from build123d import *

# Parameters (mm, degrees)
SKETCH_1_W           = 28
SKETCH_1_H           = 16
EXTRUDE_1_DEPTH      = 2
EXTRUDE_2_DEPTH      = 2
FILLET_1_R           = 3
SKETCH_3_R           = 1
CUT_EXTRUDE_1_DEPTH  = 34.526109228
EXTRUDE_3_DEPTH      = 1
EXTRUDE_3_DEPTH_BACK = 25
SKETCH_5_R           = 1
SKETCH_6_R           = 2
SKETCH_6_R_2         = 5
CUT_EXTRUDE_2_DEPTH  = 2


with BuildPart() as part:
    # Sketch 1 → Extrude 1 (new body)
    with BuildSketch(Plane(origin=(0, 0, 0), x_dir=(1, 0, 0), z_dir=(0, 1, 0))):
        Rectangle(SKETCH_1_W, SKETCH_1_H)
    extrude(amount=EXTRUDE_1_DEPTH)

    # Sketch 2 → Extrude 2 (add)
    with BuildSketch(Plane.ZY.offset(14)):
        Polygon((-8, 0), (-8, 2), (1, 12), (14, 12), (14, 6), (8, 6), (8, 2), (8, 0), align=None)
    extrude_2 = extrude(amount=-EXTRUDE_2_DEPTH)

    # Mirror 1: Extrude 2 across plane
    add(extrude_2.mirror(Plane(origin=(0, 0, 0), x_dir=(0, 0, 1), z_dir=(1, 0, 0))))

    # Fillet 1
    fillet_1_edges = [part.edges().sort_by_distance(p)[0] for p in [
        (13, 6, 14),
        (13, 12, 14),
        (-13, 6, 14),
        (-13, 12, 14),
    ]]
    fillet(fillet_1_edges, radius=FILLET_1_R - 0.0001)  # a hair under: the kernel refuses the full size

    # Sketch 3 → Cut-Extrude 1 (cut, through all)
    with BuildSketch(Plane.ZY.offset(14)):
        with Locations((11, 9)):
            Circle(SKETCH_3_R)
    extrude(amount=-CUT_EXTRUDE_1_DEPTH, mode=Mode.SUBTRACT)



with BuildPart() as body_2:
    # Sketch 4 → Revolve 2 (revolve)
    with BuildSketch(Plane(origin=(0, 9, 0), x_dir=(1, 0, 0), z_dir=(0, 1, 0))):
        with BuildLine():
            Line((-11.75, -11), (-11.75, -13.5))
            Line((-11.75, -13.5), (-3.056178347, -17.553995615))
            ThreePointArc((-3.056178347, -17.553995615), (0, -18.231534043), (3.056178347, -17.553995615))
            Line((3.056178347, -17.553995615), (11.75, -13.5))
            Line((11.75, -13.5), (11.75, -11))
            Line((11.75, -11), (-11.75, -11))
        make_face()
    revolve(axis=Axis((14, 9, 11), (-1, 0, 0)))


with BuildPart() as part_1:
    add(part.part)

    add(body_2.part)  # Extrude 3 merges body 2
    # Sketch 5 → Extrude 3 (add, two sides: drawn at the far end of the back side and taken through both)
    with BuildSketch(Plane(origin=(11.75, 0, 0), x_dir=(0, 0, -1), z_dir=(1, 0, 0)).offset(-EXTRUDE_3_DEPTH_BACK)):
        with Locations(Location((-11, 9, 0), (0, 0, 180))):
            Circle(SKETCH_5_R)
    extrude(amount=EXTRUDE_3_DEPTH + EXTRUDE_3_DEPTH_BACK)

    # Sketch 6 → Cut-Extrude 2 (cut)
    with BuildSketch(Plane.XZ):
        with Locations(Location((-8, 2, 0), (0, 0, 270))):
            Circle(SKETCH_6_R)
        with Locations(Location((8, 2, 0), (0, 0, 270))):
            Circle(SKETCH_6_R)
        with Locations(Location((0, 2, 0), (0, 0, 270))):
            Circle(SKETCH_6_R_2)
    extrude(amount=-CUT_EXTRUDE_2_DEPTH, mode=Mode.SUBTRACT)


solid = part_1.part
For this review, take the finished solid that the model builds, in its own axes (mm). A direction names the side the tool comes from. Round coordinates to 2 decimals unless told otherwise and drop trailing zeros. Loops run counter-clockwise (first coordinate to the right, second up) from the corner with the lowest first, then second, coordinate; pieces in that order, holes last. Notation, with made-up numbers: (14.5, -0.5) - (39.5, -0.5) arc R6 cw to (39.5, 9.5) - close; hole circle Ø8 at (-11.5, 45.5). An arc over 180 degrees is marked (long way). Use one line per item in the form item = value.
Item 1: For line 1 (X direction, y = 1.6, z = 2); line 2 (X direction, y = 7.75, z = 10); line 3 (X direction, y = 3, z = -5.5), list the stretches that pass through material, from the lowest coordinate up.
Answers:
line_1 = -14 to -10, -6 to -5, 5 to 6, 10 to 14
line_2 = -14 to -12, -11.75 to 11.75, 12 to 14
line_3 = -14 to -12, 12 to 14
Item 2: Consider section B-B on z = 2. Write out the cut boundary in (x, y), then the cut area to 3 significant figures.
Answers:
outline = (-14, 0) - (-10, 0) - (-10, 2) - (-12, 2) - (-12, 12) - (-14, 12) - close; (-6, 0) - (-5, 0) - (-5, 2) - (-6, 2) - close; (5, 0) - (6, 0) - (6, 2) - (5, 2) - close; (10, 0) - (14, 0) - (14, 12) - (12, 12) - (12, 2) - (10, 2) - close
area = 60.0 mm^2
Item 3: Tool access review of faces 4 (the conical face through (9.396, 6.811, 8.145)), 5 (the cylindrical face through (-12.99, 11.14, 13.1)), 6 (the cylindrical face through (12.99, 6.9, 13.14)): name each direction out of +Z, -Z, +X, -X, +Y, -Y from which nothing blocks a thin tool from reaching the whole face with its end or side.
Answers:
face_4 = none
face_5 = +Z, -X, +Y
face_6 = +Z, +X, -Y
Item 4: Consider section D-D on x = -8. Write out the cut boundary in (y, z), then the cut area to 3 significant figures.
Answers:
outline = (0, -8) - (2, -8) - (2, 0) - (0, 0) - close; (0, 4) - (2, 4) - (2, 8) - (0, 8) - close; circle Ø8.5 at (9, 11)
area = 80.7 mm^2
Item 5: Clearance check with flat-ended pins moving along their axes: P1, Ø6, axis at x = -7.5, y = 2.5, coming from the +Z side; P2, Ø4, axis at x = 8.5, y = 6, coming from the -Z side; P3, Ø1.8, axis at y = 9, z = 11, coming from the -X side. State where each tip first meets the part, or that it passes through.
Answers:
P1 = 14.41
P2 = 6.59
P3 = -13.25
Item 6: Mouldability with a two-part tool opening along X and no side actions: class faces 1 (the cylindrical face through (-4.88, 0.99, 3.08)), 2 (the flat face through (-0.2, 1.6, 8)), 3 (the flat face through (14, 6, 3)) as +X half, -X half, draft (parallel to the pull), parting line (faces both ways), or undercut.
Answers:
face_1 = undercut
face_2 = draft
face_3 = +X half
Item 7: Consider section A-A on x = 0. Write out the cut boundary in (y, z), then the cut area to 3 significant figures.
Answers:
outline = (0, -8) - (2, -8) - (2, -3) - (0, -3) - close; (0, 7) - (2, 7) - (2, 8) - (0, 8) - close; circle Ø14.46 at (9, 11)
area = 176 mm^2
Item 8: Consider section C-C on x = 5.5. Write out the cut boundary in (y, z).
Answers:
outline = (0, -8) - (2, -8) - (2, 8) - (0, 8) - close; circle Ø10.83 at (9, 11)
